```python
from build123d import *

# Parameters (mm, degrees)
SKETCH1_W               = 5.6
SKETCH1_H               = 10
BOSS_EXTRUDE1_DEPTH     = 4.5
CHAMFER1_SIZE           = 1
SKETCH2_R               = 1.5
BOSS_EXTRUDE2_DEPTH     = 0.9
SKETCH3_W               = 3.6
SKETCH3_H               = 0.5
BOSS_EXTRUDE3_DEPTH     = 2.4
CHAMFER2_SIZE           = 0.5
SKETCH4_W               = 3.5
SKETCH4_H               = 1
BOSS_EXTRUDE4_DEPTH     = 1
BOSS_EXTRUDE5_DEPTH     = 1
SKETCH6_W               = 2
SKETCH6_H               = 0.4
BOSS_EXTRUDE6_DEPTH     = 0.5
SKETCH7_W               = 0.5
SKETCH7_H               = 0.5
BOSS_EXTRUDE7_DEPTH     = 17
MIRROR3_COPY_1_SKETCH_W = 0.5
MIRROR3_COPY_1_SKETCH_H = 0.5
MIRROR3_COPY_1_DEPTH    = 17


# Read off the part's stored shape, not the designer's step: Dome1, Dome2
with BuildPart() as part:
    # Sketch1 → Boss-Extrude1 (new body)
    with BuildSketch(Plane.XY):
        Rectangle(SKETCH1_W, SKETCH1_H)
    extrude(amount=BOSS_EXTRUDE1_DEPTH)

    # Chamfer1
    chamfer1_edges = [part.edges().sort_by_distance(p)[0] for p in [
        (-2.8, 0, 4.5),
        (0, -5, 4.5),
        (2.8, 0, 4.5),
        (0, 5, 4.5),
        (2.8, -5, 2.25),
        (-2.8, -5, 2.25),
    ]]
    chamfer(chamfer1_edges, length=CHAMFER1_SIZE)

    # Sketch2 → Boss-Extrude2 (add)
    with BuildSketch(Plane.XY.offset(4.5)):
        with Locations((0, 1.85)):
            Circle(SKETCH2_R)
        with Locations((0, -1.85)):
            Circle(SKETCH2_R)
    extrude(amount=BOSS_EXTRUDE2_DEPTH)

    # Dome1 outline → Dome1 (revolve)
    with BuildSketch(Plane.XZ.offset(-1.85)):
        with BuildLine():
            Line((0, 5.4), (1.5, 5.399999999))
            ThreePointArc((1.5, 5.399999999), (1.025914227, 6.395622385), (0, 6.8))
            Line((0, 6.8), (0, 5.4))
        make_face()
    revolve(axis=Axis((0, 1.85, 0), (0, 0, 1)))

    # Dome2 outline → Dome2 (revolve)
    with BuildSketch(Plane.XZ.offset(1.85)):
        with BuildLine():
            Line((0, 5.4), (1.5, 5.399999999))
            ThreePointArc((1.5, 5.399999999), (1.025914227, 6.395622385), (0, 6.8))
            Line((0, 6.8), (0, 5.4))
        make_face()
    revolve(axis=Axis((0, -1.85, 0), (0, 0, 1)))

    # Sketch3 → Boss-Extrude3 (add)
    with BuildSketch(Plane.XY.offset(4.5)):
        Rectangle(SKETCH3_W, SKETCH3_H)
    extrude(amount=BOSS_EXTRUDE3_DEPTH)

    # Chamfer2
    chamfer2_edges = [part.edges().sort_by_distance(p)[0] for p in [
        (1.8, 0, 6.9),
        (-1.8, 0, 6.9),
    ]]
    chamfer(chamfer2_edges, length=CHAMFER2_SIZE)

    # Sketch4 → Boss-Extrude4 (add)
    with BuildSketch(Plane(origin=(2.8, 0, 0), x_dir=(0, 0, -1), z_dir=(1, 0, 0))):
        with Locations((1.75, -0.023003027)):
            Rectangle(SKETCH4_W, SKETCH4_H)
    boss_extrude4 = extrude(amount=-BOSS_EXTRUDE4_DEPTH)

    # Sketch5 → Boss-Extrude5 (add)
    with BuildSketch(Plane.XZ.offset(0.523003027)):
        Polygon((2.8, -2.633974596), (2.8, -3.5), (3.3, -2.633974596), align=None)
    boss_extrude5 = extrude(amount=-BOSS_EXTRUDE5_DEPTH)

    # Mirror1: Boss-Extrude4, Boss-Extrude5 across plane
    add(boss_extrude4.mirror(Plane(origin=(0, 0, 0), x_dir=(0, 0, 1), z_dir=(1, 0, 0))))
    add(boss_extrude5.mirror(Plane(origin=(0, 0, 0), x_dir=(0, 0, 1), z_dir=(1, 0, 0))))

    # Sketch6 → Boss-Extrude6 (add)
    with BuildSketch(Plane.ZY.offset(2.8)):
        with Locations((-1, 4.8)):
            Rectangle(SKETCH6_W, SKETCH6_H)
    extrude(amount=-BOSS_EXTRUDE6_DEPTH)

    # Sketch7 → Boss-Extrude7 (add)
    with BuildSketch(Plane(origin=(0, 0, 0), x_dir=(-1, 0, 0), z_dir=(0, 0, -1))):
        with Locations((1.3, 3)):
            Rectangle(SKETCH7_W, SKETCH7_H)
    boss_extrude7 = extrude(amount=BOSS_EXTRUDE7_DEPTH)

    # Mirror2: Boss-Extrude7 across plane
    add(boss_extrude7.mirror(Plane(origin=(0, 0, 0), x_dir=(0, 0, 1), z_dir=(1, 0, 0))))

    # Mirror3: Boss-Extrude7 across plane
    add(boss_extrude7.mirror(Plane(origin=(0, 0, 0), x_dir=(0, 0, 1), z_dir=(0, -1, 0))))

    # Mirror3 copy 1 sketch → Mirror3 copy 1 (add)
    with BuildSketch(Plane(origin=(0, 0, 0), x_dir=(1, 0, 0), z_dir=(0, 0, -1))):
        with Locations((1.3, 3)):
            Rectangle(MIRROR3_COPY_1_SKETCH_W, MIRROR3_COPY_1_SKETCH_H)
    extrude(amount=MIRROR3_COPY_1_DEPTH)


solid = part.part
```
Check sheet for the modelled part. Datum: model origin and axes. Units: mm. A direction names the side the tool comes from. Coordinates: 2 decimals unless noted, no trailing zeros. Write each loop counter-clockwise with the first axis right and the second up, starting at its lowest first coordinate (ties: lowest second). Pieces come first, ordered by that corner, then holes. Notation, with made-up numbers: M 62.5,-5 L 90.5,-5 A4 cw 90.5,-1 Z; hole C 57.25,22.5 d8. An arc over 180 degrees is marked long. Use one line per item in the form item = value.
Item 1: Sectioned sample at D-D, the plane z = 0.5. Record the cut outline in (x, y), and give its area (3 significant figures).
Answer below:
outline = M -2.8,-4 L -1.8,-5 L 1.8,-5 L 2.8,-4 L 2.8,5 L -2.8,5 Z
area = 55.0 mm^2
Item 2: Release check for a two-part mould opening along X. For faces 5 (the face through (3.05, -0.03, -3.07)), 6 (the face through (1.8, 0, -2)), 7 (the face through (2, 0, -3.5)) record: pulls with the +X half, pulls with the -X half, needs draft (parallel to the pull), parting line crosses it, or undercut.
Answer below:
face_5 = pulls with the +X half
face_6 = undercut
face_7 = needs draft
Item 3: Sectioned sample at A-A, the plane z = -5.5. Record the cut outline in (x, y).
Answer below:
outline = M -1.55,-3.25 L -1.05,-3.25 L -1.05,-2.75 L -1.55,-2.75 Z; M -1.55,2.75 L -1.05,2.75 L -1.05,3.25 L -1.55,3.25 Z; M 1.05,-3.25 L 1.55,-3.25 L 1.55,-2.75 L 1.05,-2.75 Z; M 1.05,2.75 L 1.55,2.75 L 1.55,3.25 L 1.05,3.25 Z
Item 4: Sectioned sample at B-B, the plane y = -1.85. Record the cut outline in (x, z).
Answer below:
outline = M -2.8,0 L 2.8,0 L 2.8,3.5 L 1.8,4.5 L 1.5,4.5 L 1.5,5.4 A1.5 ccw -1.5,5.4 L -1.5,4.5 L -1.8,4.5 L -2.8,3.5 Z
Item 5: Set-up check for faces 1 (the face through (-2.8, 1, 2)), 2 (the face through (-1.5, 1.9, 4.9)), 3 (the face through (-2, -0.523, -2)), 4 (the face through (-1.8, 0, -2)): record each of +Z, -Z, +X, -X, +Y, -Y from which the full face is reachable in a straight line by a thin tool's end or side.
Answer below:
face_1 = +Z, -X, +Y, -Y
face_2 = +Z
face_3 = -Z, +X, -X, -Y
face_4 = -Z, +Y, -Y
Item 6: Gauge pin test, flat ends, axial feed: pin 1 Ø1.8 at (x, y) = (1, 2) entering from +Z; pin 2 Ø0.5 at (x, y) = (-2, 0) entering from -Z; pin 3 Ø1.2 at (x, z) = (-0.5, 5.5) entering from -Y. Record the tip position at first contact, or that the pin passes through.
Answer below:
pin_1 = 6.8
pin_2 = -3.5
pin_3 = -3.35
Item 7: Material ranges on L1, parallel to X at y = -3, z = -2.5; L2, parallel to Y at x = -1.5, z = -12.25; L3, parallel to Y at x = -2.5, z = -0.75, recorded low to high. Write a range as from..to.
Answer below:
L1 = -1.55..-1.05, 1.05..1.55
L2 = -3.25..-2.75, 2.75..3.25
L3 = -0.52..0.48, 4.6..5
